Can you work these out from the model? Positions are in its coordinate system, mm. Give positions to 0.01 mm unless a question says otherwise; leave off trailing zeros. Order: outer loops, then holes, each group sorted by start corner. A loop starts at its lowest first (then second) coordinate and runs counter-clockwise, first axis right, second up.
Item 1: If we mould it in two halves opening along Y, with no side actions, what happens to faces 1 (the flat face through (25, 0, 99)), 2 (the flat face through (0, 25, 99)), 3 (the cylindrical face through (0.4, -12.4, 28.2))? For each: +Y half, -Y half, draft (parallel to the pull), parting line (faces both ways), or undercut.
Item 2: I want a section at A-A, the plane y = -10. Write out the boundary of the cut face in (x, z), then the cut area to 3 significant figures.
Item 3: If I drill on line 1 along Y through (x, z) = (9.5, 175), over which ranges is the centre line in solid material (lowest first)?
Item 4: I want a section at B-B, the plane z = 25. Write out the boundary of the cut face in (x, y).
Autodesk Inventor part; units mm, degrees
ref_plane "YZ Plane" through (0, 0, 0) normal (1, 0, 0) x (0, 1, 0)
ref_plane "XZ Plane" through (0, 0, 0) normal (0, 1, 0) x (-1, 0, 0)
ref_plane "XY Plane" through (0, 0, 0) normal (0, 0, 1) x (1, 0, 0)
sketch "Sketch1" plane through (0, 0, 0) normal (0, 0, 1) x (1, 0, 0)
  line L0 (25, -25) -> (-25, -25)
  line L1 (-25, -25) -> (-25, 25)
  line L2 (-25, 25) -> (25, 25)
  line L3 (25, 25) -> (25, -25)
  line L4 (25, -25) -> (-25, 25) construction
  line L5 (-25, -25) -> (25, 25) construction
  point P0 (0, 0)
  dimension "d0" = 50
  dimension "d1" = 50
extrude "Extrusion1" add sketch "Sketch1" along normal blind 200
sketch "Sketch2" plane through (25, -25, 0) normal (1, 0, 0) x (0, 0, -1)
  circle A0 centre (-175, 15) radius 4
  circle A1 centre (-25, 15) radius 4
  line L0 (0, 0) -> (-200, 0)
  line L1 (-200, 0) -> (-200, 50)
  point P0 (0, 25)
  dimension "d4" = 8
  dimension "d5" = 15
  dimension "d6" = 8
  dimension "d7" = 15
  dimension "d8" = 25
  dimension "d9" = 25
extrude "Extrusion2" cut sketch "Sketch2" against normal through all
properties part number "Blok_roda"
Results list:
1. face 1: draft
1. face 2: +Y half
1. face 3: undercut
2. outline: (-25, 0) - (25, 0) - (25, 21) - (-25, 21) - close; (-25, 29) - (25, 29) - (25, 171) - (-25, 171) - close; (-25, 179) - (25, 179) - (25, 200) - (-25, 200) - close
2. area: 9,200 mm2
3. line 1: y = -25 to -14, -6 to 25
4. outline: (-25, -25) - (25, -25) - (25, -14) - (-25, -14) - close; (-25, -6) - (25, -6) - (25, 25) - (-25, 25) - close
